The model under review builds one solid part; all positions refer to its coordinate system, in mm. A direction names the side the tool comes from. Coordinates: 2 decimals unless noted, no trailing zeros. Write each loop counter-clockwise with the first axis right and the second up, starting at its lowest first coordinate (ties: lowest second). Pieces come first, ordered by that corner, then holes. Notation, with made-up numbers: (64.25, -8) - (120.25, -8) arc R30 cw to (120.25, 27) - close; hole circle Ø1 at (-1.75, 28.25). An arc over 180 degrees is marked (long way). Return JSON: item names as keys, results as strings. Group by question number.
(1) We need section A-A on y = 2.75. State the section outline as (x, z) points.
(2) Draft analysis for pull direction X (two halves, no side actions). For faces 4 (the face through (-10.5, 6.3, 11.3)), 5 (the face through (6, 6, 18.896)), 6 (the face through (71.55, 6.26, -6.01)), state which applies: released by +X, released by -X, zero draft, split by the parting line, or undercut.
(3) We need section B-B on x = 55. State the section outline as (y, z) points, then the cut area to 3 significant figures.
(4) For pin 1 Ø4 at (x, y) = (7, 8) entering from +Z; pin 2 Ø4 at (x, y) = (58.5, 7) entering from +Z; pin 3 Ø1 at (x, y) = (49, 7.5) entering from +Z; pin 4 Ø5 at (x, z) = (22.44, 11.77) entering from +Y, all flat-tipped, find the tip position at first contact; note any pin that passes through.
(5) We need section C-C on z = 16.5. State the section outline as (x, y) points.
(6) To check wall thickness, follow L1, parallel to Z at x = -8.5, y = 6.25; L2, parallel to X at y = 9.5, z = 3; L3, parallel to Z at x = -18, y = 8. State the ranges of each line that lie inside material, in increasing order. Write a range as from..to.
(7) Tool access review of faces 1 (the face through (-12.554, 6.261, -3.39)), 2 (the face through (61, 6, -6.254)), 3 (the face through (25, 0, 6)): name each direction out of +Z, -Z, +X, -X, +Y, -Y from which nothing blocks a thin tool from reaching the whole face with its end or side.
```python
from build123d import *

# Parameters (mm, degrees)
SKETCH1_R           = 3.2639
BOSS_EXTRUDE1_DEPTH = 12.7


with BuildPart() as part:
    # Sketch1 → Boss-Extrude1 (new body)
    with BuildSketch(Plane(origin=(0, 0, 0), x_dir=(1, 0, 0), z_dir=(0, 1, 0))):
        with BuildLine():
            Line((-8.873253367, 0), (45.204292469, 0))
            ThreePointArc((45.204292469, 0), (46.502747155, 0.356971043), (47.436232768, 1.327546907))
            Line((47.436232768, 1.327546907), (49.391348597, 4.926615465))
            ThreePointArc((49.391348597, 4.926615465), (50.324834209, 5.897191329), (51.623288895, 6.254162372))
            Line((51.623288895, 6.254162372), (70.462087223, 6.254162372))
            ThreePointArc((70.462087223, 6.254162372), (71.559520533, 6.004847887), (72.441516032, 5.305847513))
            Line((72.441516032, 5.305847513), (76.972410672, -0.328799158))
            ThreePointArc((76.972410672, -0.328799158), (56.487992256, -17.897771795), (30.865519551, -26.369435729))
            Line((30.865519551, -26.369435729), (18.165519551, -18.896027316))
            Line((18.165519551, -18.896027316), (-5.688817186, -18.896027316))
            ThreePointArc((-5.688817186, -18.896027316), (-18.253794481, -13.20459823), (-29.23375861, -4.855262498))
            Line((-29.23375861, -4.855262498), (-29.23375861, 4.177286104))
            ThreePointArc((-29.23375861, 4.177286104), (-28.489809834, 5.973337328), (-26.69375861, 6.717286104))
            Line((-26.69375861, 6.717286104), (-16.191261416, 6.717286104))
            ThreePointArc((-16.191261416, 6.717286104), (-15.013419953, 6.427683732), (-14.10416564, 5.624915621))
            Line((-14.10416564, 5.624915621), (-10.960349143, 1.092370482))
            ThreePointArc((-10.960349143, 1.092370482), (-10.05109483, 0.289602371), (-8.873253367, 0))
        make_face()
        with Locations((-20.368787798, -1.624222444)):
            Circle(SKETCH1_R, mode=Mode.SUBTRACT)
        with Locations((-7.908365266, -9.317144856)):
            Circle(SKETCH1_R, mode=Mode.SUBTRACT)
        with Locations((7.107001098, -10.503835127)):
            Circle(SKETCH1_R, mode=Mode.SUBTRACT)
        with Locations((22.444824189, -11.767482364)):
            Circle(SKETCH1_R, mode=Mode.SUBTRACT)
    extrude(amount=BOSS_EXTRUDE1_DEPTH)


solid = part.part
```
Ans:
{
 "1": {"outline": "(-29.23, -4.18) arc R2.54 ccw to (-26.69, -6.72) - (-16.19, -6.72) arc R2.54 ccw to (-14.1, -5.62) - (-10.96, -1.09) arc R2.54 cw to (-8.87, 0) - (45.2, 0) arc R2.54 cw to (47.44, -1.33) - (49.39, -4.93) arc R2.54 ccw to (51.62, -6.25) - (70.46, -6.25) arc R2.54 ccw to (72.44, -5.31) - (76.97, 0.33) arc R69.71 ccw to (30.87, 26.37) - (18.17, 18.9) - (-5.69, 18.9) arc R61.48 ccw to (-29.23, 4.86) - close; hole circle Ø6.53 at (-20.37, 1.62); hole circle Ø6.53 at (-7.91, 9.32); hole circle Ø6.53 at (7.11, 10.5); hole circle Ø6.53 at (22.44, 11.77)"},
 "2": {"face 4": "undercut", "face 5": "zero draft", "face 6": "released by +X"},
 "3": {"outline": "(0, -6.25) - (12.7, -6.25) - (12.7, 18.71) - (0, 18.71) - close", "area": "317 mm²"},
 "4": {"pin 1": "z = 18.9", "pin 2": "z = 17.89", "pin 3": "z = 21.76", "pin 4": "through"},
 "5": {"outline": "(-11.92, 0) - (58.85, 0) - (58.85, 12.7) - (-11.92, 12.7) - close"},
 "6": {"L1": "0..6.11, 12.53..17.91", "L2": "-29.23..-23.33, -17.41..74.76", "L3": "-6.72..-0.62, 3.87..13.36"},
 "7": {"face 1": "-Z, +Y, -Y", "face 2": "-Z, +X, +Y, -Y", "face 3": "+Z, -Z, +X, -X, -Y"}
}
